```python
from build123d import *

# Parameters (mm, degrees)
F1_DEPTH = 50.8
F2_START = -12.7
F0_R     = 1.3146247551
F2_DEPTH = 12.7
F3_START = 12.7
F3_DEPTH = 12.7
F4_SIZE  = 5.08


with BuildPart() as f1:
    # F0 (on Front) → F1 (new body, symmetric)
    with BuildSketch(Plane.XZ):
        Polygon((90.658403933, 5.5023488702), (-7.2033622317, 5.5023488702), (-7.2033622317, 1.6923488702), (145.1966377683, 1.6923488702), (145.1966377683, 5.5023488702), align=None)
    extrude(amount=F1_DEPTH, both=True)

    # F0 (on Front) → F2 (join)
    with BuildSketch(Plane.XZ.offset(F2_START)):
        Polygon((90.658403933, 5.5023488702), (-7.2033622317, 5.5023488702), (-7.2033622317, 1.6923488702), (145.1966377683, 1.6923488702), (145.1966377683, 5.5023488702), align=None)
        with BuildLine():
            Line((90.658403933, 24.540095979), (90.658403933, 5.5023488702))
            Line((90.658403933, 5.5023488702), (145.1966377683, 5.5023488702))
            Line((145.1966377683, 5.5023488702), (145.1966377683, 27.080095979))
            Line((145.1966377683, 27.080095979), (93.198403933, 27.080095979))
            ThreePointArc((93.198403933, 27.080095979), (91.4023527088, 26.3361472032), (90.658403933, 24.540095979))
        make_face()
        with Locations((93.198403933, 24.540095979)):
            Circle(F0_R, mode=Mode.SUBTRACT)
    extrude(amount=-F2_DEPTH)

    # F0 (on Front) → F3 (join)
    with BuildSketch(Plane.XZ.offset(F3_START)):
        Polygon((90.658403933, 5.5023488702), (-7.2033622317, 5.5023488702), (-7.2033622317, 1.6923488702), (145.1966377683, 1.6923488702), (145.1966377683, 5.5023488702), align=None)
        with BuildLine():
            Line((90.658403933, 24.540095979), (90.658403933, 5.5023488702))
            Line((90.658403933, 5.5023488702), (145.1966377683, 5.5023488702))
            Line((145.1966377683, 5.5023488702), (145.1966377683, 27.080095979))
            Line((145.1966377683, 27.080095979), (93.198403933, 27.080095979))
            ThreePointArc((93.198403933, 27.080095979), (91.4023527088, 26.3361472032), (90.658403933, 24.540095979))
        make_face()
        with Locations((93.198403933, 24.540095979)):
            Circle(F0_R, mode=Mode.SUBTRACT)
    extrude(amount=F3_DEPTH)

    # F4
    f4_edges = [f1.edges().sort_by_distance(p)[0] for p in [
        (145.196638, 19.05, 27.080096),
        (145.196638, -19.05, 27.080096),
    ]]
    chamfer(f4_edges, length=F4_SIZE)


solid = f1.part
```
Check sheet for the modelled part. Datum: model origin and axes. Units: mm. A direction names the side the tool comes from. Round coordinates to 2 decimals unless told otherwise and drop trailing zeros. Order: outer loops, then holes, each group sorted by start corner. A loop starts at its lowest first (then second) coordinate and runs counter-clockwise, first axis right, second up. Notation, with made-up numbers: (-36, 56.5) -> (-19, 56.5) arc R10 cw to (-19, 74.5) -> close; hole circle Ø7 at (45.5, -36). An arc over 180 degrees is marked (long way). One line per item, written item: value. Start each with the question number.
Q1. Cross-section at A-A (z = 7.5). Record the boundary of the cut face in (x, y), and give its area (3 significant figures).
Q2. Set-up check for faces 1 (the face through (90.658, -19, 15)), 2 (the face through (142.621, -18.961, 24.576)), 3 (the face through (118, 25.4, 16)): record each of +Z, -Z, +X, -X, +Y, -Y from which the full face is reachable in a straight line by a thin tool's end or side.
Q3. Mould release check, pull along Y, two halves, no side actions. Record for faces 4 (the face through (118, -12.7, 16)), 5 (the face through (118, -25.4, 16)), 6 (the face through (118, 12.7, 16)), 7 (the face through (145.197, -1, 5)): pulls with the +Y half, pulls with the -Y half, needs draft (parallel to the pull), parting line crosses it, or undercut.
Q4. Cross-section at B-B (y = -19). Record the boundary of the cut face in (x, z), and give its area (3 significant figures).
Q5. Thickness scan on line 1 (Y direction, x = 117.5, z = 25.75); line 2 (Z direction, x = 57.5, y = 25); line 3 (X direction, y = 14, z = 15.25). Record the ranges inside material, lowest first.
Q6. Cross-section at C-C (x = 9). Record the boundary of the cut face in (y, z), and give its area (3 significant figures).
Q7. Cross-section at D-D (y = -33). Record the boundary of the cut face in (x, z), and give its area (3 significant figures).
Q8. Gauge pin test, flat ends, axial feed: pin 1 Ø4 at (x, z) = (65.5, 6.5) entering from +Y; pin 2 Ø6 at (x, z) = (89.5, 16) entering from +Y; pin 3 Ø1.5 at (x, y) = (29, -11.5) entering from +Z; pin 4 Ø10 at (y, z) = (21.5, 12.5) entering from -X. Record the tip position at first contact, or that the pin passes through.
Completed:
1. outline: (90.66, -25.4) -> (145.2, -25.4) -> (145.2, -12.7) -> (90.66, -12.7) -> close; (90.66, 12.7) -> (145.2, 12.7) -> (145.2, 25.4) -> (90.66, 25.4) -> close
1. area: 1,390 mm²
2. face 1: +Z, -X, +Y, -Y
2. face 2: +Z, +X, +Y, -Y
2. face 3: +Z, +X, -X, +Y
3. face 4: undercut
3. face 5: pulls with the -Y half
3. face 6: undercut
3. face 7: needs draft
4. outline: (-7.2, 1.69) -> (145.2, 1.69) -> (145.2, 22) -> (140.12, 27.08) -> (93.2, 27.08) arc R2.54 ccw to (90.66, 24.54) -> (90.66, 5.5) -> (-7.2, 5.5) -> close; hole circle Ø2.63 at (93.2, 24.54)
4. area: 1,740 mm²
5. line 1: y = -25.4 to -12.7, 12.7 to 25.4
5. line 2: z = 1.69 to 5.5
5. line 3: x = 90.66 to 145.2
6. outline: (-50.8, 1.69) -> (50.8, 1.69) -> (50.8, 5.5) -> (-50.8, 5.5) -> close
6. area: 387 mm²
7. outline: (-7.2, 1.69) -> (145.2, 1.69) -> (145.2, 5.5) -> (-7.2, 5.5) -> close
7. area: 581 mm²
8. pin 1: stops at y = 50.8
8. pin 2: stops at y = 25.4
8. pin 3: stops at z = 5.5
8. pin 4: stops at x = 90.66
